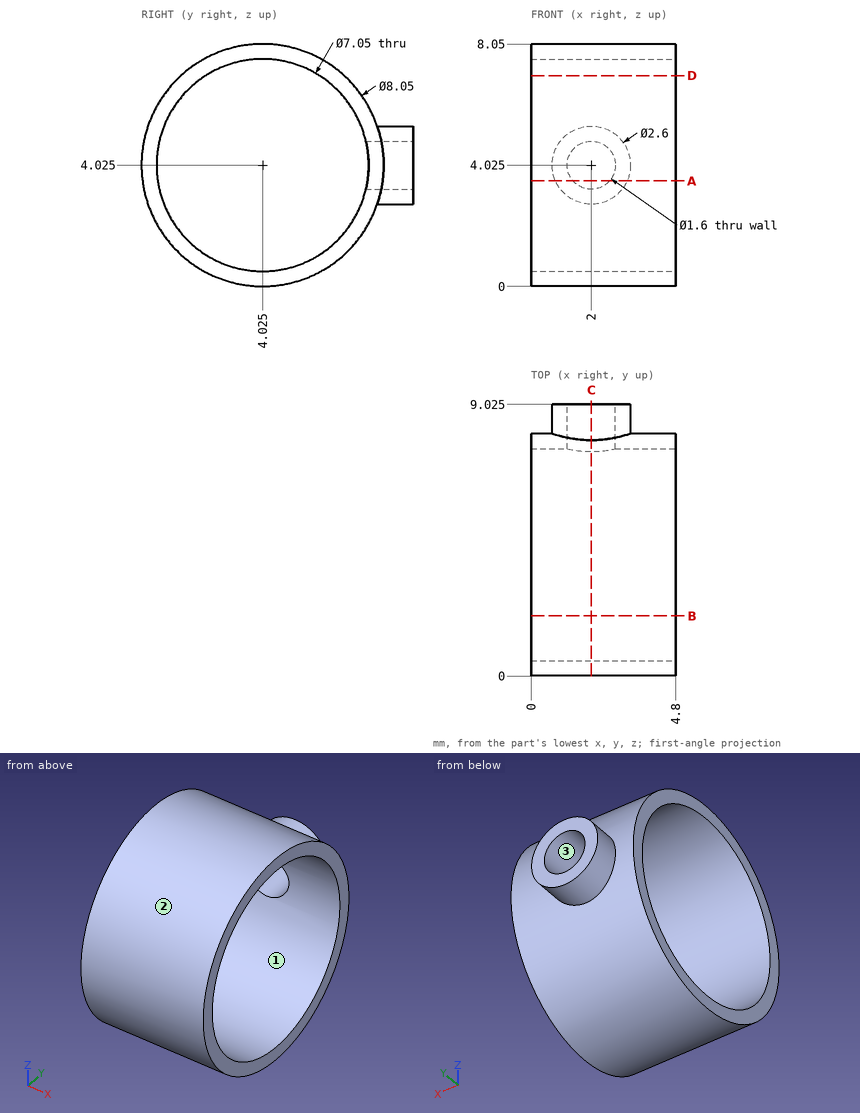
Geometry check sheet. Reference: drawing and pictorial views, mm from the part's lowest x, y, z. Round coordinates to 2 decimals unless told otherwise and drop trailing zeros. Order: outer loops, then holes, each group sorted by start corner. A loop starts at its lowest first (then second) coordinate and runs counter-clockwise, first axis right, second up. Notation, with made-up numbers: (55.5, 53.5) - (97.5, 53.5) arc R16 ccw to (97.5, 81.5) - close; hole circle Ø1 at (77, 66.25). An arc over 180 degrees is marked (long way). Use a Markdown table: item, result. Add a question column.
1) Mould release check, pull along Y, two halves, no side actions. Record for the marked faces 1, 2 and 3: released by +Y, released by -Y, zero draft, split by the parting line, or undercut.
2) Gauge pin test, flat end, axial feed: P1, Ø2, axis at x = 1.5, z = 5.5, coming from the -Y side. Record the tip position at first contact, or that the pin passes through.
3) Section check B-B (y = 2). Record the cut outline in (x, z).
4) Section check D-D (z = 7). Record the cut outline in (x, y).
5) Section check A-A (z = 3.5). Record the cut outline in (x, y) (3 decimals), then the cut area to 3 significant figures.
6) Section check C-C (x = 2). Record the cut outline in (y, z) (3 decimals), then the cut area to 3 significant figures.
7) Thickness scan on line 1 along Z through (x, y) = (2, 8.5) (3 decimals); line 2 along Y through (x, z) = (3.9, 4.5); line 3 along Y through (x, z) = (0.5, 1). Record the ranges inside material, lowest first.
Established:
| question | item | result |
|---|---|---|
| 1 | face 1 | undercut |
| 1 | face 2 | split by the parting line |
| 1 | face 3 | zero draft |
| 2 | P1 | y = 0.03 |
| 3 | outline | (0, 0.55) - (4.8, 0.55) - (4.8, 1.14) - (0, 1.14) - close; (0, 6.91) - (4.8, 6.91) - (4.8, 7.5) - (0, 7.5) - close |
| 4 | outline | (0, 1.31) - (4.8, 1.31) - (4.8, 2.13) - (0, 2.13) - close; (0, 5.92) - (4.8, 5.92) - (4.8, 6.74) - (0, 6.74) - close |
| 5 | outline | (0, 0.034) - (4.8, 0.034) - (4.8, 0.539) - (0, 0.539) - close; (0, 7.511) - (1.396, 7.511) - (1.396, 9.025) - (0.811, 9.025) - (0.811, 8.016) - (0, 8.016) - close; (2.604, 7.511) - (4.8, 7.511) - (4.8, 8.016) - (3.189, 8.016) - (3.189, 9.025) - (2.604, 9.025) - close |
| 5 | area | 5.42 mm2 |
| 6 | outline | (7.458, 3.225) arc R3.525 cw (long way) to (7.458, 4.825) - (9.025, 4.825) - (9.025, 5.325) - (7.834, 5.325) arc R4.025 ccw (long way) to (7.834, 2.725) - (9.025, 2.725) - (9.025, 3.225) - close |
| 6 | area | 12.2 mm2 |
| 7 | line 1 | 2.725 to 3.225, 4.825 to 5.325 |
| 7 | line 2 | 0.03 to 0.53, 7.52 to 8.02 |
| 7 | line 3 | 1.37 to 2.22, 5.83 to 6.68 |
